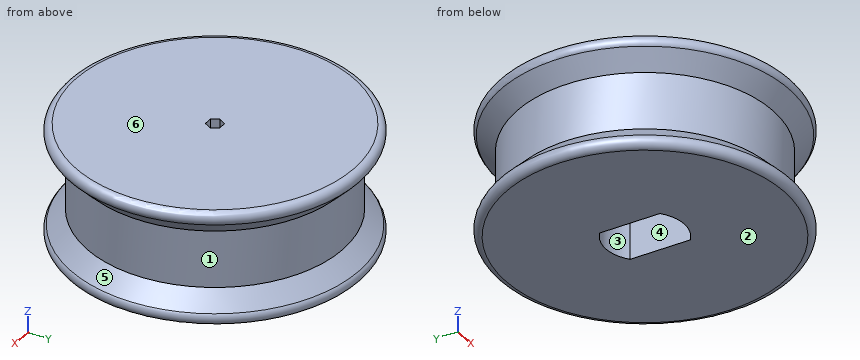
Autodesk Inventor part; units mm, degrees
ref_plane "YZ Plane" through (0, 0, 0) normal (1, 0, 0) x (0, 1, 0)
ref_plane "XZ Plane" through (0, 0, 0) normal (0, 1, 0) x (-1, 0, 0)
ref_plane "XY Plane" through (0, 0, 0) normal (0, 0, 1) x (1, 0, 0)
sketch "Sketch1" plane through (0, 0, 0) normal (0, 0, 1) x (1, 0, 0)
  line L0 (1.5, -2) -> (1.5, 2)
  line L1 (-1.5, 2) -> (-1.5, -2)
  arc A0 (-1.5, -2) -> (1.5, -2) centre (0, 0) ccw
  arc A1 (1.5, 2) -> (-1.5, 2) centre (0, 0) ccw
  line L2 (-1.75, 2.1213) -> (-1.75, -2.1213)
  arc A2 (-1.75, -2.1213) -> (1.75, -2.1213) centre (0, 0) ccw
  line L3 (1.75, -2.1213) -> (1.75, 2.1213)
  arc A3 (1.75, 2.1213) -> (-1.75, 2.1213) centre (0, 0) ccw
  circle A4 centre (0, 0) radius 11
  dimension "d0" = 3
  dimension "d2" = 2.5
  dimension "d3" = 0.25
  dimension "d4" = 22
extrude "Extrusion1" add sketch "Sketch1" along normal blind 6 contours A4
sketch "Sketch2" plane through (0, 0, 6) normal (0, 0, 1) x (1, 0, 0)
  circle A0 centre (0, 0) radius 11
extrude "Extrusion2" add sketch "Sketch2" along normal blind 2
sketch "Sketch3" plane through (0, 0, 8) normal (0, 0, 1) x (1, 0, 0)
  line L0 (0.5774, 0) -> (0.2887, -0.5)
  line L1 (0.2887, -0.5) -> (-0.2887, -0.5)
  line L2 (-0.2887, -0.5) -> (-0.5774, 0)
  line L3 (-0.5774, 0) -> (-0.2887, 0.5)
  line L4 (-0.2887, 0.5) -> (0.2887, 0.5)
  line L5 (0.2887, 0.5) -> (0.5774, 0)
  point P0 (0, 0)
  point P1 (0, 0)
  dimension "d24" = 1
sketch "Sketch4" plane through (0, 0, 0) normal (1, 0, 0) x (0, 1, 0)
  line L0 (11, 8) -> (-11, 8)
  line L1 (-11, 0) -> (11, 0)
  line L2 (11, 8) -> (11, 0)
  line L3 (11, 0) -> (9, 2)
  line L4 (9, 2) -> (9, 6)
  line L5 (9, 6) -> (11, 8)
  line L6 (0, -1.6) -> (0, 9.6)
  point P0 (0, 0)
  dimension "d16" = 45
  dimension "d17" = 45
  dimension "d18" = 4
revolve "Revolution1" cut sketch "Sketch4" angle 360 about axis through (0, 0, -10) along (0, 0, 1) contours L2 L3 L4 L5
fillet "Fillet1" radius 0.5 2 edges at (0, -11, 0) (0, -11, 8)
extrude "Extrusion3" cut sketch "Sketch3" against normal through all
properties part number "22mm Spool" material "ABS Plastic"
CAD build for the part. Positions are in the model's coordinates, mm. Face numbers are marked on the shaded views. A direction names the side the tool comes from. Coordinates: 2 decimals unless noted, no trailing zeros. Write each loop counter-clockwise with the first axis right and the second up, starting at its lowest first coordinate (ties: lowest second). Pieces come first, ordered by that corner, then holes. Notation, with made-up numbers: (3, -19.75) -> (52, -19.75) arc R17 ccw to (52, -13.75) -> close; hole circle Ø1 at (-20.5, 50.25). An arc over 180 degrees is marked (long way). Return JSON: item names as keys, results as strings. Group by question number.
Q1. Cut at C-C, the plane z = 2.25. Give the cut face in (x, y).
Q2. Cut at B-B, the plane x = 0. Give the cut face in (y, z), then the cut area to 3 significant figures.
Q3. Drill centre lines: line 1 (X direction, y = -0.25, z = 1.5); line 2 (X direction, y = 1, z = 0.5); line 3 (Z direction, x = -4.25, y = 8.25). Where is each one in solid material? Low to high.
Q4. Flat gauge pins, fed straight in: pin 1 (1.5 mm diameter, centred on y = 1.5, z = 1, fed in from +X); pin 2 (1.5 mm diameter, centred on x = -5.5, z = 6, fed in from +Y); pin 3 (3 mm diameter, centred on x = 0, z = 5, fed in from +Y). Where does each tip first touch, or does it go through?
Q5. Cut at A-A, the plane z = 6.25. Give the cut face in (x, y), then the cut area to 3 significant figures.
Q6. Which spindle directions (+Z, -Z, +X, -X, +Y, -Y) get a long thin tool onto all of the face, cutting with end or side? Do the marked faces 5 and 6. Say none if no direction does.
Q7. Pull direction Y, two halves, no side cores. Call the marked faces 1, 2, 3 and 4: released by +Y, released by -Y, zero draft, split by the parting line, or undercut.
Returned:
{
 "1": {"outline": "circle Ø18 at (0, 0); hole (-1.75, -2.12) arc R2.75 ccw to (1.75, -2.12) -> (1.75, 2.12) arc R2.75 ccw to (-1.75, 2.12) -> close"},
 "2": {"outline": "(-10.15, 0.85) arc R0.5 ccw to (-9.79, 0) -> (-2.75, 0) -> (-2.75, 6) -> (-0.5, 6) -> (-0.5, 8) -> (-9.79, 8) arc R0.5 ccw to (-10.15, 7.15) -> (-9, 6) -> (-9, 2) -> close; (0.5, 6) -> (2.75, 6) -> (2.75, 0) -> (9.79, 0) arc R0.5 ccw to (10.15, 0.85) -> (9, 2) -> (9, 6) -> (10.15, 7.15) arc R0.5 ccw to (9.79, 8) -> (0.5, 8) -> close", "area": "116 mm2"},
 "3": {"line 1": "x = -9.5 to -1.75, 1.75 to 9.5", "line 2": "x = -10.24 to -1.75, 1.75 to 10.24", "line 3": "z = 0 to 1.72, 6.28 to 8"},
 "4": {"pin 1": "stops at x = 10.25", "pin 2": "stops at y = 8.18", "pin 3": "stops at y = 9.5"},
 "5": {"outline": "circle Ø18.5 at (0, 0); hole (-0.58, 0) -> (-0.29, -0.5) -> (0.29, -0.5) -> (0.58, 0) -> (0.29, 0.5) -> (-0.29, 0.5) -> close", "area": "268 mm2"},
 "6": {"face 5": "none", "face 6": "+Z, +X, -X, +Y, -Y"},
 "7": {"face 1": "split by the parting line", "face 2": "zero draft", "face 3": "undercut", "face 4": "undercut"}
}
